from build123d import *

# Parameters (mm, degrees)
BOSS_EXTRUDE1_DEPTH        = 1.5
F_3_2_3_2_DIAMETER_HOLE1_D = 3.2


with BuildPart() as part:
    # Sketch1 → Boss-Extrude1 (new body)
    with BuildSketch(Plane(origin=(0, 0, 0), x_dir=(1, 0, 0), z_dir=(0, 1, 0))):
        with BuildLine():
            Line((-18.944019139, 12.822966507), (16.455980861, 12.822966507))
            ThreePointArc((16.455980861, 12.822966507), (18.082326458, 12.149312104), (18.755980861, 10.522966507))
            Line((18.755980861, 10.522966507), (18.755980861, -24.877033493))
            ThreePointArc((18.755980861, -24.877033493), (18.082326458, -26.50337909), (16.455980861, -27.177033493))
            ThreePointArc((16.455980861, -27.177033493), (14.829635265, -26.50337909), (14.155980861, -24.877033493))
            Line((14.155980861, -24.877033493), (14.155980861, -24.733717149))
            ThreePointArc((14.155980861, -24.733717149), (13.482326458, -23.107371553), (11.855980861, -22.433717149))
            Line((11.855980861, -22.433717149), (-14.344019139, -22.433717149))
            ThreePointArc((-14.344019139, -22.433717149), (-15.970364735, -23.107371553), (-16.644019139, -24.733717149))
            Line((-16.644019139, -24.733717149), (-16.644019139, -24.877033493))
            ThreePointArc((-16.644019139, -24.877033493), (-17.317673542, -26.50337909), (-18.944019139, -27.177033493))
            ThreePointArc((-18.944019139, -27.177033493), (-20.570364735, -26.50337909), (-21.244019139, -24.877033493))
            Line((-21.244019139, -24.877033493), (-21.244019139, 10.522966507))
            ThreePointArc((-21.244019139, 10.522966507), (-20.570364735, 12.149312104), (-18.944019139, 12.822966507))
        make_face()
    extrude(amount=BOSS_EXTRUDE1_DEPTH)

    # Ø3.2 (3.2) Diameter Hole1 (through all)
    with Locations(Plane(origin=(0, 1.5, 0), x_dir=(1, 0, 0), z_dir=(0, 1, 0))):
        with Locations((-18.944019139, 10.522966507), (16.455980861, 10.522966507), (16.455980861, -24.877033493), (-18.944019139, -24.877033493)):
            Hole(F_3_2_3_2_DIAMETER_HOLE1_D / 2)


solid = part.part
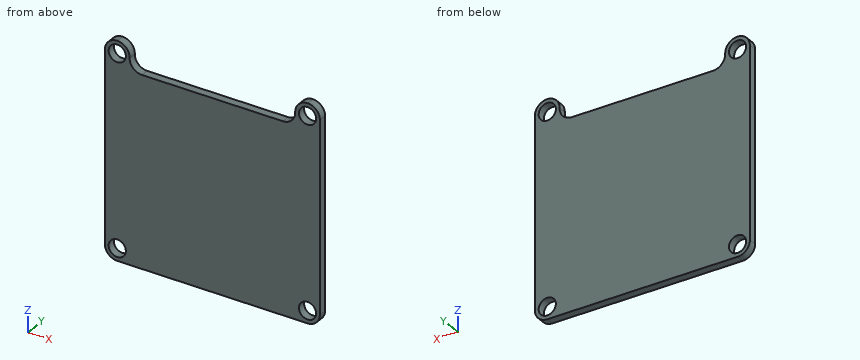
Build history of the part. All positions in model axes, mm. Coordinates: 2 decimals unless noted, no trailing zeros. Order: outer loops, then holes, each group sorted by start corner. A loop starts at its lowest first (then second) coordinate and runs counter-clockwise, first axis right, second up. Notation, with made-up numbers: M -38,-26 L -33,-26 A24 ccw -33,1 Z; hole C 60.5,18 d11. An arc over 180 degrees is marked long. One line per question, with ' | ' between items. Start each with the question number.
Q1. Saw through at B-B (x = 13). List the corners of the cut face in (y, z), then the cut area to 3 significant figures.
Q2. Probe L1, parallel to Z at x = -19, y = 0.7; L2, parallel to Z at x = -13, y = 0.1; L3, parallel to X at y = 0.95, z = -9.5. List the from-to ranges inside material, lowest first. Write a range as from..to.
Q3. Saw through at C-C (x = -0.5). List the corners of the cut face in (y, z), then the cut area to 3 significant figures.
Q4. Saw through at A-A (y = 0.55). List the corners of the cut face in (x, z).
Check values:
1) outline: M 0,-12.82 L 1.5,-12.82 L 1.5,22.74 L 0,22.74 Z | area: 53.3 mm2
2) L1: z = -12.82..-12.12, -8.92..23.28, 26.48..27.18 | L2: z = -12.82..22.43 | L3: x = -21.24..-20.17, -17.71..15.23, 17.69..18.76
3) outline: M 0,-12.82 L 1.5,-12.82 L 1.5,22.43 L 0,22.43 Z | area: 52.9 mm2
4) outline: M -21.24,-10.52 A2.3 ccw -18.94,-12.82 L 16.46,-12.82 A2.3 ccw 18.76,-10.52 L 18.76,24.88 A2.3 ccw 14.16,24.88 L 14.16,24.73 A2.3 cw 11.86,22.43 L -14.34,22.43 A2.3 cw -16.64,24.73 L -16.64,24.88 A2.3 ccw -21.24,24.88 Z; hole C -18.94,-10.52 d3.2; hole C -18.94,24.88 d3.2; hole C 16.46,-10.52 d3.2; hole C 16.46,24.88 d3.2
